from build123d import *

# Parameters (mm, degrees)
SKETCH1_R           = 132
BOSS_EXTRUDE1_DEPTH = 5
SKETCH2_R           = 132
SKETCH2_R_2         = 128
BOSS_EXTRUDE2_DEPTH = 25
SKETCH3_R           = 25
BOSS_EXTRUDE3_DEPTH = 25
SKETCH4_W           = 24.259702766
SKETCH4_H           = 53.634785552
CUT_EXTRUDE1_DEPTH  = 25
SKETCH5_W           = 53.321862162
SKETCH5_H           = 77.08657154
SKETCH5_W_2         = 44.150486072
SKETCH5_H_2         = 70.031666854
CUT_EXTRUDE2_DEPTH  = 25
SKETCH6_W           = 57.100495662
SKETCH6_H           = 46.822548266
SKETCH6_W_2         = 44.150486072
SKETCH6_H_2         = 23.467734864
CUT_EXTRUDE4_DEPTH  = 25
SKETCH7_R           = 5
CUT_EXTRUDE5_DEPTH  = 60
SKETCH8_R           = 6
CUT_EXTRUDE6_DEPTH  = 30
BOSS_EXTRUDE4_START = -5
SKETCH9_R           = 5
BOSS_EXTRUDE4_DEPTH = 5
CIRPATTERN1_COUNT   = 4


with BuildPart() as part:
    # Sketch1 → Boss-Extrude1 (new body)
    with BuildSketch(Plane.XY):
        Circle(SKETCH1_R)
    extrude(amount=BOSS_EXTRUDE1_DEPTH)

    # Sketch2 → Boss-Extrude2 (add)
    with BuildSketch(Plane.XY.offset(5)):
        Circle(SKETCH2_R)
        Circle(SKETCH2_R_2, mode=Mode.SUBTRACT)
    extrude(amount=BOSS_EXTRUDE2_DEPTH)

    # Sketch3 → Boss-Extrude3 (add)
    with BuildSketch(Plane.XY.offset(5)):
        Circle(SKETCH3_R)
    extrude(amount=BOSS_EXTRUDE3_DEPTH)

    # Sketch4 → Cut-Extrude1 (cut)
    with BuildSketch(Plane.XY.offset(30)):
        Rectangle(SKETCH4_W, SKETCH4_H)
    extrude(amount=-CUT_EXTRUDE1_DEPTH, mode=Mode.SUBTRACT)

    # Sketch5 → Cut-Extrude2 (cut)
    with BuildSketch(Plane.XY.offset(30)):
        Rectangle(SKETCH5_W, SKETCH5_H)
        Rectangle(SKETCH5_W_2, SKETCH5_H_2, mode=Mode.SUBTRACT)
    extrude(amount=-CUT_EXTRUDE2_DEPTH, mode=Mode.SUBTRACT)

    # Sketch6 → Cut-Extrude4 (cut)
    with BuildSketch(Plane.XY.offset(30)):
        Rectangle(SKETCH6_W, SKETCH6_H)
        Rectangle(SKETCH6_W_2, SKETCH6_H_2, mode=Mode.SUBTRACT)
    extrude(amount=-CUT_EXTRUDE4_DEPTH, mode=Mode.SUBTRACT)

    # Sketch7 → Cut-Extrude5 (cut)
    with BuildSketch(Plane(origin=(22.075243036, 0, 0), x_dir=(0, 0, -1), z_dir=(1, 0, 0))):
        with Locations((-15, 0)):
            Circle(SKETCH7_R)
    extrude(amount=-CUT_EXTRUDE5_DEPTH, mode=Mode.SUBTRACT)

    # Sketch8 → Cut-Extrude6 (cut, symmetric)
    with BuildSketch(Plane.XY.offset(5)):
        Circle(SKETCH8_R)
    extrude(amount=CUT_EXTRUDE6_DEPTH, both=True, mode=Mode.SUBTRACT)

    # Sketch9 → Boss-Extrude4 (add)
    with BuildSketch(Plane.XY.offset(30).offset(BOSS_EXTRUDE4_START)):
        with BuildLine():
            ThreePointArc((-129.632575758, -24.887653615), (-132, 0), (-129.632575758, 24.887653615))
            ThreePointArc((-129.632575758, 24.887653615), (-157, 0), (-129.632575758, -24.887653615))
        make_face()
        with Locations((-144.000711393, 0)):
            Circle(SKETCH9_R, mode=Mode.SUBTRACT)
    boss_extrude4 = extrude(amount=BOSS_EXTRUDE4_DEPTH)

    # CirPattern1: Boss-Extrude4 ×4 about axis
    cirpattern1_axis = Axis((0, 0, 0), (0, 0, 1))
    for i in range(1, CIRPATTERN1_COUNT):
        add(boss_extrude4.rotate(cirpattern1_axis, i * 360 / CIRPATTERN1_COUNT))


solid = part.part
The model under review builds one solid part; all positions refer to its coordinate system, in mm. A direction names the side the tool comes from. Give positions to 0.01 mm unless a question says otherwise; leave off trailing zeros. Write each loop counter-clockwise with the first axis right and the second up, starting at its lowest first coordinate (ties: lowest second). Pieces come first, ordered by that corner, then holes.
1. For P1, Ø8, axis at x = 98.5, z = 24.5, coming from the -Y side; P2, Ø13.5, axis at x = -5, y = 146, coming from the -Z side; P3, Ø8, axis at x = -7.5, y = 90.5, coming from the +Z side; P4, Ø11.5, axis at y = 2, z = 23, coming from the -X side, all flat-tipped, find the tip position at first contact; note any pin that passes through.
2. Wall thickness on L1, parallel to X at y = 3.5, z = 11.25; L2, parallel to Y at x = 0, z = 23.5; L3, parallel to Y at x = 20, z = 8.5: over which ranges is each line inside the solid? List them lowest first.
3. Add section A-A, the plane z = 15. Write out the cut boundary in (x, y).
4. Add section C-C, the plane y = 86. Write out the cut boundary in (x, z), plus the area to 3 significant figures.
5. Draft analysis for pull direction X (two halves, no side actions). For faces 5 (the cylindrical face through (-0.583, -156.993, 27.465)), 6 (the cylindrical face through (-27.748, -124.956, 17.325)), 7 (the flat face through (-2, -27, 0)), state which applies: +X half, -X half, draft (parallel to the pull), parting line (faces both ways), or undercut.
6. Add section D-D, the plane x = 85.5. Write out the cut boundary in (y, z), plus the area to 3 significant figures.
7. Tool access review of faces 1 (the cylindrical face through (-6, 0, 3)), 2 (the cylindrical face through (-17, 0, 20)), 3 (the flat face through (22.075, -0.2, 20.5)), 4 (the cylindrical face through (121.934, -50.557, 14.79)): name each direction out of +Z, -Z, +X, -X, +Y, -Y from which nothing blocks a thin tool from reaching the whole face with its end or side.
8. Add section B-B, the plane x = 0. Write out the cut boundary in (y, z), plus the area to 3 significant figures.
Worked answers:
1. P1: stops at y = -92.16
1. P2: stops at z = 25
1. P3: stops at z = 5
1. P4: stops at x = -157
2. L1: x = -131.95 to -127.95, -22.08 to -12.13, 12.13 to 22.08, 127.95 to 131.95
2. L2: y = -132 to -128, 128 to 132
2. L3: y = -130.48 to -126.43, -11.73 to 11.73, 126.43 to 130.48
3. outline: circle Ø264 at (0, 0); (-22.08, -11.73) - (-12.13, -11.73) - (-12.13, -5) - (-22.08, -5) - close; (-22.08, 5) - (-12.13, 5) - (-12.13, 11.73) - (-22.08, 11.73) - close; (12.13, -11.73) - (22.08, -11.73) - (22.08, -5) - (12.13, -5) - close; (12.13, 5) - (22.08, 5) - (22.08, 11.73) - (12.13, 11.73) - close; hole circle Ø256 at (0, 0)
4. outline: (-100.14, 0) - (100.14, 0) - (100.14, 30) - (94.81, 30) - (94.81, 5) - (-94.81, 5) - (-94.81, 30) - (-100.14, 30) - close
4. area: 1,270 mm2
5. face 5: parting line
5. face 6: undercut
5. face 7: draft
6. outline: (-100.57, 0) - (100.57, 0) - (100.57, 30) - (95.26, 30) - (95.26, 5) - (-95.26, 5) - (-95.26, 30) - (-100.57, 30) - close
6. area: 1,270 mm2
7. face 1: +Z, -Z
7. face 2: none
7. face 3: +Z
7. face 4: -Z
8. outline: (-157, 25) - (-149, 25) - (-149, 30) - (-157, 30) - close; (-139, 25) - (-132, 25) - (-132, 0) - (-6, 0) - (-6, 5) - (-128, 5) - (-128, 30) - (-139, 30) - close; (6, 0) - (132, 0) - (132, 25) - (139, 25) - (139, 30) - (128, 30) - (128, 5) - (6, 5) - close; (149, 25) - (157, 25) - (157, 30) - (149, 30) - close
8. area: 1,610 mm2
